The drawing under review shows one solid part. Ordinate dimensions are in mm from its lowest x, y, z. Coordinates: 2 decimals unless noted, no trailing zeros. Write each loop counter-clockwise with the first axis right and the second up, starting at its lowest first coordinate (ties: lowest second). Pieces come first, ordered by that corner, then holes.
Q1. Mouldability with a two-part tool opening along Z and no side actions: class the marked faces 1 and 2 as pulls with the +Z half, pulls with the -Z half, needs draft (parallel to the pull), parting line crosses it, or undercut.
Q2. Take a section at D-D (z = 0.65). Give the boundary of the cut face in (x, y).
Q3. Take a section at A-A (y = 15.5). Give the boundary of the cut face in (x, z), and give its area (3 significant figures).
Q4. Insertion check: pin 1 (2 mm diameter, centred on x = 37, y = 12.5, fed in from +Z). The pin has a flat end and moves straight along its axis. Give the tip position at first contact, or say it passes through.
Q5. Take a section at B-B (x = 25.5). Give the boundary of the cut face in (y, z).
Q6. Take a section at C-C (y = 6). Give the boundary of the cut face in (x, z).
Q7. For probe 1 along X at (y, z) = (13, 2.65); probe 2 along X at (y, z) = (6, 0.1); probe 3 along Y at (x, z) = (39, 0.25), list the stretches that pass through material, from the lowest coordinate up.
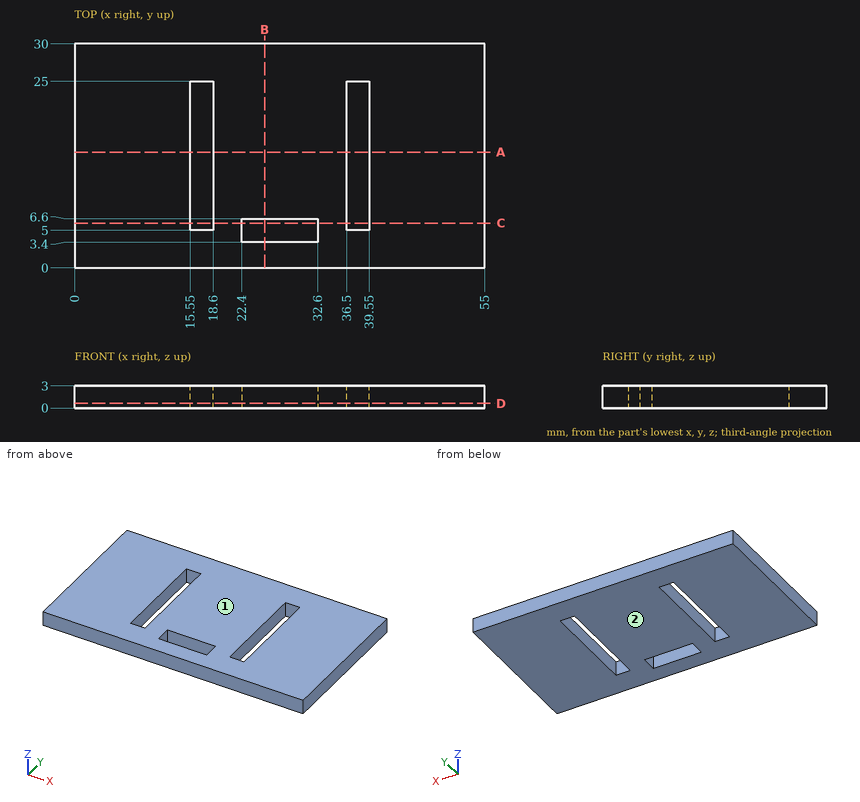
Response:
1. face 1: pulls with the +Z half
1. face 2: pulls with the -Z half
2. outline: (0, 0) - (55, 0) - (55, 30) - (0, 30) - close; hole (15.55, 5) - (18.6, 5) - (18.6, 25) - (15.55, 25) - close; hole (22.4, 3.4) - (32.6, 3.4) - (32.6, 6.6) - (22.4, 6.6) - close; hole (36.5, 5) - (39.55, 5) - (39.55, 25) - (36.5, 25) - close
3. outline: (0, 0) - (15.55, 0) - (15.55, 3) - (0, 3) - close; (18.6, 0) - (36.5, 0) - (36.5, 3) - (18.6, 3) - close; (39.55, 0) - (55, 0) - (55, 3) - (39.55, 3) - close
3. area: 147 mm2
4. pin 1: stops at z = 3
5. outline: (0, 0) - (3.4, 0) - (3.4, 3) - (0, 3) - close; (6.6, 0) - (30, 0) - (30, 3) - (6.6, 3) - close
6. outline: (0, 0) - (15.55, 0) - (15.55, 3) - (0, 3) - close; (18.6, 0) - (22.4, 0) - (22.4, 3) - (18.6, 3) - close; (32.6, 0) - (36.5, 0) - (36.5, 3) - (32.6, 3) - close; (39.55, 0) - (55, 0) - (55, 3) - (39.55, 3) - close
7. probe 1: x = 0 to 15.55, 18.6 to 36.5, 39.55 to 55
7. probe 2: x = 0 to 15.55, 18.6 to 22.4, 32.6 to 36.5, 39.55 to 55
7. probe 3: y = 0 to 5, 25 to 30
